```python
from build123d import *

# Parameters (mm, degrees)
SZKIC1_R                    = 11.115
DODANIE_WYCI_GNI_CIE1_DEPTH = 90
SFAZOWANIE1_SIZE            = 1
WYTNIJ_WYCI_GNI_CIE1_DEPTH  = 36
ZAOKR_GLENIE1_R             = 2.39
ZAOKR_GLENIE2_R             = 2.39


with BuildPart() as part:
    # Szkic1 → Dodanie-wyciągnięcie1 (new body)
    with BuildSketch(Plane.XY):
        with Locations(Location((0, 0, 0), (0, 0, 180))):
            Circle(SZKIC1_R)
    extrude(amount=DODANIE_WYCI_GNI_CIE1_DEPTH)

    # Sfazowanie1
    sfazowanie1_edges = [part.edges().sort_by_distance(p)[0] for p in [
        (11.115, 0, 0),
    ]]
    chamfer(sfazowanie1_edges, length=SFAZOWANIE1_SIZE)

    # Szkic2 → Wytnij-wyciągnięcie1 (cut)
    with BuildSketch(Plane(origin=(0, 0, 6), x_dir=(-1, 0, 0), z_dir=(0, 0, -1))):
        with BuildLine():
            Line((-2.39, 10.855004606), (-2.39, 8.465004606))
            Line((-2.39, 8.465004606), (2.39, 8.465004606))
            Line((2.39, 8.465004606), (2.39, 10.855004606))
            ThreePointArc((2.39, 10.855004606), (0, 11.115), (-2.39, 10.855004606))
        make_face()
    extrude(amount=-WYTNIJ_WYCI_GNI_CIE1_DEPTH, mode=Mode.SUBTRACT)

    # Zaokrąglenie1
    zaokr_glenie1_edges = [part.edges().sort_by_distance(p)[0] for p in [
        (-2.39, 9.660004606, 42),
        (2.39, 9.660004606, 42),
    ]]
    fillet(zaokr_glenie1_edges, radius=ZAOKR_GLENIE1_R - 0.0001)  # a hair under: the kernel refuses the full size

    # Zaokrąglenie2
    zaokr_glenie2_edges = [part.edges().sort_by_distance(p)[0] for p in [
        (2.39, 9.660004606, 6),
        (-2.39, 9.660004606, 6),
    ]]
    fillet(zaokr_glenie2_edges, radius=ZAOKR_GLENIE2_R - 0.0001)  # a hair under: the kernel refuses the full size


solid = part.part
```
Verification items for the finished model (mm, model axes). A direction names the side the tool comes from. Round coordinates to 2 decimals unless told otherwise and drop trailing zeros. Write each loop counter-clockwise with the first axis right and the second up, starting at its lowest first coordinate (ties: lowest second). Pieces come first, ordered by that corner, then holes.
1. Gauge pin test, flat ends, axial feed: P1, Ø0.7, axis at y = 9.5, z = 31, coming from the -X side; P2, Ø10, axis at x = -7.5, z = 46.5, coming from the +Y side; P3, Ø2.5, axis at y = 9.5, z = 27, coming from the +X side. Record the tip position at first contact, or that the pin passes through.
2. Access from +Z, -Z, +X, -X, +Y, -Y to the whole of each face (thin tool, end or side, straight path). Record for faces 5 (the cylindrical face through (-10.6, -3.34, 44.88)), 6 (the cylindrical face through (-1.67, 9.81, 6.68)).
3. Draft check along Z on faces 1 (the cylindrical face through (-1.67, 9.81, 41.32)), 2 (the flat face through (0, 0, 0)), 3 (the flat face through (0, 0, 90)), 4 (the cylindrical face through (1.71, 9.77, 41.28)). Enter one of: +Z half, -Z half, draft (parallel to the pull), parting line (faces both ways), or undercut.
4. Section check A-A on z = 70. Enter the section's corners in (x, y) (3 decimals).
5. Section check B-B on z = 10. Enter the section's corners in (x, y) (3 decimals).
6. Scan lines: L1, parallel to Y at x = -0.25, z = 5.5; L2, parallel to X at y = -7.25, z = 38 (3 decimals); L3, parallel to X at y = -1.5, z = 64.5. Record each from-to range of solid material in increasing order.
Answer:
1. P1: stops at x = -6.31
1. P2: stops at y = 10.83
1. P3: stops at x = 7.45
2. face 5: +Z, -Z
2. face 6: +Y
3. face 1: undercut
3. face 2: -Z half
3. face 3: +Z half
3. face 4: undercut
4. outline: circle Ø22.23 at (0, 0)
5. outline: (-2.39, 8.465) - (-2.39, 10.855) arc R11.115 ccw (long way) to (2.39, 10.855) - (2.39, 8.465) - close
6. L1: y = -11.11 to 11.11
6. L2: x = -8.425 to 8.425
6. L3: x = -11.01 to 11.01
